Read the model definition and answer for the solid it produces. Units are mm, in the model's axes. A direction names the side the tool comes from. Coordinates: 2 decimals unless noted, no trailing zeros. Loops run counter-clockwise (first coordinate to the right, second up) from the corner with the lowest first, then second, coordinate; pieces in that order, holes last. Notation, with made-up numbers: M 49.5,58.5 L 61.5,58.5 A8 cw 61.5,66.5 Z; hole C 29,74 d10. An arc over 180 degrees is marked long. One line per item, written item: value. Start each with the question number.
```python
from build123d import *

# Parameters (mm, degrees)
SKETCH1_W           = 139.5
SKETCH1_H           = 152.4
BOSS_EXTRUDE1_DEPTH = 6.35
SKETCH2_W           = 139.5
SKETCH2_H           = 152.4
CUT_EXTRUDE1_DEPTH  = 3.375
SKETCH3_R           = 2.286
BOSS_EXTRUDE2_DEPTH = 12.7
SKETCH4_R           = 2.286
BOSS_EXTRUDE3_DEPTH = 12.7


with BuildPart() as part:
    # Sketch1 → Boss-Extrude1 (new body)
    with BuildSketch(Plane(origin=(0, 0, 0), x_dir=(1, 0, 0), z_dir=(0, 1, 0))):
        with Locations((69.75, 76.2)):
            Rectangle(SKETCH1_W, SKETCH1_H)
    extrude(amount=BOSS_EXTRUDE1_DEPTH)

    # Sketch2 → Cut-Extrude1 (cut)
    with BuildSketch(Plane(origin=(0, 6.35, 0), x_dir=(1, 0, 0), z_dir=(0, 1, 0))):
        with Locations((69.75, 76.2)):
            Rectangle(SKETCH2_W, SKETCH2_H)
    extrude(amount=-CUT_EXTRUDE1_DEPTH, mode=Mode.SUBTRACT)

    # Sketch3 → Boss-Extrude2 (add)
    with BuildSketch(Plane.XY):
        with BuildLine():
            Line((63.4, 9.325), (63.4, 2.975))
            Line((63.4, 2.975), (76.1, 2.975))
            Line((76.1, 2.975), (76.1, 9.325000158))
            ThreePointArc((76.1, 9.325000158), (69.749999921, 15.675000158), (63.4, 9.325))
        make_face()
        with Locations((69.75, 9.325000158)):
            Circle(SKETCH3_R, mode=Mode.SUBTRACT)
    extrude(amount=-BOSS_EXTRUDE2_DEPTH)

    # Sketch4 → Boss-Extrude3 (add)
    with BuildSketch(Plane(origin=(0, 0, -152.4), x_dir=(-1, 0, 0), z_dir=(0, 0, -1))):
        with BuildLine():
            Line((-130.61, 9.325), (-130.61, 2.975))
            Line((-130.61, 2.975), (-117.91, 2.975))
            Line((-117.91, 2.975), (-117.91, 9.325))
            ThreePointArc((-117.91, 9.325), (-124.26, 15.675), (-130.61, 9.325))
        make_face()
        with Locations((-124.26, 9.325)):
            Circle(SKETCH4_R, mode=Mode.SUBTRACT)
        with BuildLine():
            Line((-21.59, 9.325), (-21.59, 2.975))
            Line((-21.59, 2.975), (-8.89, 2.975))
            Line((-8.89, 2.975), (-8.89, 9.325))
            ThreePointArc((-8.89, 9.325), (-15.24, 15.675), (-21.59, 9.325))
        make_face()
        with Locations((-15.24, 9.325)):
            Circle(SKETCH4_R, mode=Mode.SUBTRACT)
    extrude(amount=-BOSS_EXTRUDE3_DEPTH)


solid = part.part
```
1) Flat-ended cylindrical pins translate along their axes: pin 1 (6 mm diameter, centred on x = 58.5, y = 9, fed in from -Z); pin 2 (6 mm diameter, centred on x = 124.26, y = 9.325, fed in from +Z); pin 3 (12 mm diameter, centred on x = 87.5, z = -21.5, fed in from +Y) (3 decimals); pin 4 (5 mm diameter, centred on y = 7.5, z = -5, fed in from +X). Find the tip coordinate at first contact, or state that the pin passes through.
2) Section B-B (y = 4.75) is taken. Determine the outline of the cut face in (x, z).
3) Consider line 1 along Y through (x, z) = (124.26, -146) (3 decimals); line 2 along Y through (x, z) = (124, -145); line 3 along Z through (x, y) = (21, 11). Determine where each line is inside the solid, lowest interval first.
4) A tool of negligible diameter and unlimited length cuts with its end or side. For faces 4 (the face through (15.3, 6.6, -139.7)), 5 (the face through (8.89, 6, -146)), 6 (the face through (76.1, 6, -6)), from which of +Z, -Z, +X, -X, +Y, -Y can it reach the whole face along a straight path? Write none if from no direction.
5) Section A-A (x = 69.75) is taken. Determine the outline of the cut face in (y, z) (3 decimals).
6) Section D-D (y = 13.75) is taken. Determine the outline of the cut face in (x, z), then the cut area to 3 significant figures.
7) Section C-C (z = -51) is taken. Determine the outline of the cut face in (x, y) (3 decimals), then the cut area to 3 significant figures.
8) For a pull along Y with two mould halves and no side action, classify faces 1 (the face through (124.3, 6.6, -139.7)), 2 (the face through (13.13, 8.45, -146.14)), 3 (the face through (69.89, 15.673, -6.261)) as released by +Y, released by -Y, zero draft, split by the parting line, or undercut.
Results found:
1. pin 1: passes through
1. pin 2: stops at z = -139.7
1. pin 3: stops at y = 2.975
1. pin 4: stops at x = 76.1
2. outline: M 8.89,-152.4 L 21.59,-152.4 L 21.59,-139.7 L 8.89,-139.7 Z; M 63.4,-12.7 L 76.1,-12.7 L 76.1,0 L 63.4,0 Z; M 117.91,-152.4 L 130.61,-152.4 L 130.61,-139.7 L 117.91,-139.7 Z
3. line 1: y = 0 to 7.039, 11.611 to 15.675
3. line 2: y = 0 to 7.05, 11.6 to 15.67
3. line 3: z = -152.4 to -139.7
4. face 4: +Z, +X, -X, +Y
4. face 5: +Z, -Z, -X, +Y
4. face 6: +Z, -Z, +X, +Y
5. outline: M 0,-152.4 L 2.975,-152.4 L 2.975,-12.7 L 7.039,-12.7 L 7.039,0 L 0,0 Z; M 11.611,-12.7 L 15.675,-12.7 L 15.675,0 L 11.611,0 Z
6. outline: M 10.69,-152.4 L 19.79,-152.4 L 19.79,-139.7 L 10.69,-139.7 Z; M 65.2,-12.7 L 74.3,-12.7 L 74.3,0 L 65.2,0 Z; M 119.71,-152.4 L 128.81,-152.4 L 128.81,-139.7 L 119.71,-139.7 Z
6. area: 347 mm²
7. outline: M 0,0 L 139.5,0 L 139.5,2.975 L 0,2.975 Z
7. area: 415 mm²
8. face 1: zero draft
8. face 2: undercut
8. face 3: released by +Y
